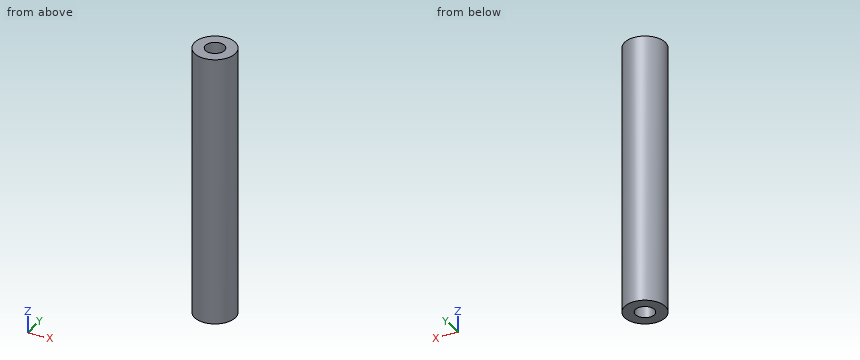
Autodesk Inventor part; units mm, degrees
ref_plane "YZ Plane" through (0, 0, 0) normal (1, 0, 0) x (0, 1, 0)
ref_plane "XZ Plane" through (0, 0, 0) normal (0, 1, 0) x (-1, 0, 0)
ref_plane "XY Plane" through (0, 0, 0) normal (0, 0, 1) x (1, 0, 0)
sketch "スケッチ1" plane through (0, 0, 0) normal (0, 0, 1) x (1, 0, 0)
  circle A0 centre (0, 0) radius 1.4
  circle A1 centre (0, 0) radius 3
  dimension "d0" = 2.8
  dimension "d1" = 6
extrude "押し出し1" add sketch "スケッチ1" along normal blind 40 contours A0 | A1
sketch "スケッチ2" plane through (0, 0, 40) normal (0, 0, 1) x (1, 0, 0)
  circle A0 centre (0, 0) radius 1.4
  dimension "d4" = 2.8
extrude "押し出し2" cut sketch "スケッチ2" against normal blind 6
extrude "押し出し3" cut sketch "スケッチ1" along normal blind 6 contours A0
properties part number "40mm" material "アルミニウム 2014-T4"
The model under review builds one solid part; all positions refer to its coordinate system, in mm. Round coordinates to 2 decimals unless told otherwise and drop trailing zeros. Write each loop counter-clockwise with the first axis right and the second up, starting at its lowest first coordinate (ties: lowest second). Pieces come first, ordered by that corner, then holes. Notation, with made-up numbers: (16.25, -25.75) - (43.25, -25.75) arc R22 cw to (43.25, 9.25) - close; hole circle Ø6 at (20.5, -30). An arc over 180 degrees is marked (long way). Answer as CSV lines item,"result". Start each with the question number.
(1) We need section D-D on z = 19.5. State the section outline as (x, y) points, plus the area to 3 significant figures.
(2) To check wall thickness, follow line 1 (Y direction, x = 0, z = 2.2); line 2 (X direction, y = 0.3, z = 35); line 3 (Z direction, x = 0.95, y = 0.3). State the ranges of each line that lie inside material, in increasing order.
(3) We need section A-A on y = 0. State the section outline as (x, z) points, plus the area to 3 significant figures.
(4) For pin 1 Ø0.8 at (x, y) = (0.5, 0) entering from +Z; pin 2 Ø1.5 at (y, z) = (-2, 27) entering from +X; pin 3 Ø1.7 at (x, y) = (0, 0) entering from -Z, all flat-tipped, find the tip position at first contact; note any pin that passes through.
(5) We need section C-C on z = 4. State the section outline as (x, y) points, plus the area to 3 significant figures.
Worked answers:
1,outline,"circle Ø6 at (0, 0)"
1,area,"28.3 mm²"
2,line 1,"-3 to -1.4, 1.4 to 3"
2,line 2,"-2.98 to -1.37, 1.37 to 2.98"
2,line 3,"6 to 34"
3,outline,"(-3, 0) - (-1.4, 0) - (-1.4, 6) - (1.4, 6) - (1.4, 0) - (3, 0) - (3, 40) - (1.4, 40) - (1.4, 34) - (-1.4, 34) - (-1.4, 40) - (-3, 40) - close"
3,area,"206 mm²"
4,pin 1,"z = 34"
4,pin 2,"x = 2.73"
4,pin 3,"z = 6"
5,outline,"circle Ø6 at (0, 0); hole circle Ø2.8 at (0, 0)"
5,area,"22.1 mm²"
